Source: CAD feature listing. Evaluate the final solid. Frame: model axes, mm. Give positions to 0.01 mm unless a question says otherwise; leave off trailing zeros. Loops run counter-clockwise (first coordinate to the right, second up) from the corner with the lowest first, then second, coordinate; pieces in that order, holes last. Notation, with made-up numbers: M 66.5,41 L 78.5,41 A15 ccw 78.5,55 Z; hole C -1,-40 d1. An arc over 180 degrees is marked long. Write item = value, one per line.
from build123d import *

# Parameters (mm, degrees)
MODEL_R         = 1
EXTRUDE_1_DEPTH = 1.2


with BuildPart() as part:
    # Model → 凸台-拉伸1 (new body)
    with BuildSketch(Plane.XY):
        with BuildLine():
            ThreePointArc((12.485683382, 19.826470809), (12.652302696, 19.686300725), (12.828649886, 19.55858496))
            ThreePointArc((12.828649886, 19.55858496), (15.184787498, 18.84198425), (17.540925109, 19.55858496))
            ThreePointArc((17.540925109, 19.55858496), (17.7172723, 19.686300725), (17.883891613, 19.826470809))
            ThreePointArc((17.883891613, 19.826470809), (21.053773782, 19.747678625), (21.132565966, 16.577796457))
            ThreePointArc((21.132565966, 16.577796457), (20.992395882, 16.411177143), (20.864680117, 16.234829953))
            ThreePointArc((20.864680117, 16.234829953), (20.148079407, 13.878692341), (20.864680117, 11.522554729))
            ThreePointArc((20.864680117, 11.522554729), (20.992395882, 11.346207539), (21.132565966, 11.179588225))
            ThreePointArc((21.132565966, 11.179588225), (21.053773782, 8.009706057), (17.883891613, 7.930913873))
            ThreePointArc((17.883891613, 7.930913873), (17.7172723, 8.071083957), (17.540925109, 8.198799722))
            ThreePointArc((17.540925109, 8.198799722), (15.184787498, 8.915400432), (12.828649886, 8.198799722))
            ThreePointArc((12.828649886, 8.198799722), (12.652302696, 8.071083957), (12.485683382, 7.930913873))
            ThreePointArc((12.485683382, 7.930913873), (9.315801214, 8.009706057), (9.237009029, 11.179588225))
            ThreePointArc((9.237009029, 11.179588225), (9.377179113, 11.346207539), (9.504894878, 11.522554729))
            ThreePointArc((9.504894878, 11.522554729), (10.221495588, 13.878692341), (9.504894878, 16.234829953))
            ThreePointArc((9.504894878, 16.234829953), (9.377179113, 16.411177143), (9.237009029, 16.577796457))
            ThreePointArc((9.237009029, 16.577796457), (9.315801214, 19.747678625), (12.485683382, 19.826470809))
        make_face()
        with Locations((18.296057335, 16.989962178)):
            Circle(MODEL_R, mode=Mode.SUBTRACT)
        with Locations((12.07351766, 16.989962178)):
            Circle(MODEL_R, mode=Mode.SUBTRACT)
        with Locations((12.07351766, 10.767422504)):
            Circle(MODEL_R, mode=Mode.SUBTRACT)
        with Locations((18.296057335, 10.767422504)):
            Circle(MODEL_R, mode=Mode.SUBTRACT)
    extrude(amount=EXTRUDE_1_DEPTH)


solid = part.part
1. Material intervals for probe 1 along X at (y, z) = (16.5, 0.6); probe 2 along X at (y, z) = (10.75, 0.35); probe 3 along Y at (x, z) = (18, 0.1), sorted ascending. Write a range as from..to.
Derived:
probe_1 = 9.31..11.2, 12.95..17.42, 19.17..21.06
probe_2 = 8.93..11.07, 13.07..17.3, 19.3..21.44
probe_3 = 7.83..9.81, 11.72..16.03, 17.95..19.92
2. Pull-direction query (Y, two-part tool) for faces 1 (the cylindrical face through (15.15, 18.842, 0.592)), 2 (the cylindrical face through (15.22, 8.915, 0.592)), 3 (the flat face through (15, 14, 1.2)), 4 (the cylindrical face through (19.22, 16.61, 0.59)); classes: +Y half, -Y half, draft (parallel to the pull), parting line (faces both ways), or undercut.
Derived:
face_1 = +Y half
face_2 = -Y half
face_3 = draft
face_4 = undercut
3. Cut plane A-A, the plane x = 9.75. Return the cut outline in (y, z).
Derived:
outline = M 7.67,0 L 11.94,0 L 11.94,1.2 L 7.67,1.2 Z; M 15.82,0 L 20.09,0 L 20.09,1.2 L 15.82,1.2 Z
4. Cut plane C-C, the plane x = 18.5. Return the cut outline in (y, z).
Derived:
outline = M 7.53,0 L 9.79,0 L 9.79,1.2 L 7.53,1.2 Z; M 11.75,0 L 16.01,0 L 16.01,1.2 L 11.75,1.2 Z; M 17.97,0 L 20.23,0 L 20.23,1.2 L 17.97,1.2 Z
5. Cut plane D-D, the plane z = 0.55. Return the cut outline in (x, y), then the cut area to 3 significant figures.
Derived:
outline = M 9.24,11.18 A2.3 ccw 12.49,7.93 A3 cw 12.83,8.2 A4.23 cw 17.54,8.2 A3 cw 17.88,7.93 A2.3 ccw 21.13,11.18 A3 cw 20.86,11.52 A4.23 cw 20.86,16.23 A3 cw 21.13,16.58 A2.3 ccw 17.88,19.83 A3 cw 17.54,19.56 A4.23 cw 12.83,19.56 A3 cw 12.49,19.83 A2.3 ccw 9.24,16.58 A3 cw 9.5,16.23 A4.23 cw 9.5,11.52 A3 cw Z; hole C 12.07,10.77 d2; hole C 12.07,16.99 d2; hole C 18.3,10.77 d2; hole C 18.3,16.99 d2
area = 124 mm²
6. Cut plane B-B, the plane y = 10.5. Return the cut outline in (x, z).
Derived:
outline = M 8.81,0 L 11.11,0 L 11.11,1.2 L 8.81,1.2 Z; M 13.04,0 L 17.33,0 L 17.33,1.2 L 13.04,1.2 Z; M 19.26,0 L 21.56,0 L 21.56,1.2 L 19.26,1.2 Z
